Autodesk Inventor part; units mm, degrees
ref_plane "YZ Plane" through (0, 0, 0) normal (1, 0, 0) x (0, 1, 0)
ref_plane "XZ Plane" through (0, 0, 0) normal (0, 1, 0) x (-1, 0, 0)
ref_plane "XY Plane" through (0, 0, 0) normal (0, 0, 1) x (1, 0, 0)
sketch "Sketch1" plane through (0, 0, 0) normal (0, 1, 0) x (-1, 0, 0)
  line L0 (52.5, 37) -> (-52.5, 37)
  line L1 (-54.5, 35) -> (-54.5, -35)
  line L2 (-52.5, -37) -> (52.5, -37)
  line L3 (54.5, -35) -> (54.5, 35)
  line L4 (54.5, 37) -> (-54.5, -37) construction
  line L5 (-54.5, 37) -> (54.5, -37) construction
  circle A0 centre (-40.5, -31) radius 2.15
  circle A1 centre (-40.5, 31) radius 2.15
  circle A2 centre (9.5, -31) radius 2.15
  circle A3 centre (9.5, 31) radius 2.15
  circle A4 centre (32.1, 26) radius 2.15
  circle A5 centre (32.1, -26) radius 2.15
  circle A6 centre (9.6, 12.319) radius 3.95
  circle A7 centre (9.6, -12.319) radius 3.95
  circle A8 centre (-40.4, 12.319) radius 3.95
  circle A9 centre (-40.4, -12.319) radius 3.95
  circle A10 centre (43.1, 19.95) radius 3.95
  circle A11 centre (43.1, -19.95) radius 3.95
  arc A12 (54.5, 35) -> (52.5, 37) centre (52.5, 35) ccw
  arc A13 (52.5, -37) -> (54.5, -35) centre (52.5, -35) ccw
  arc A14 (-54.5, -35) -> (-52.5, -37) centre (-52.5, -35) ccw
  arc A15 (-52.5, 37) -> (-54.5, 35) centre (-52.5, 35) ccw
  circle A16 centre (44.5, -7.5) radius 2
  circle A17 centre (44.5, 7.5) radius 2
  point P0 (0, 0)
  dimension "d0" = 109
  dimension "d1" = 74
  dimension "d2" = 4.3
  dimension "d3" = 6
  dimension "d4" = 14
  dimension "d5" = 4.3
  dimension "d6" = 6
  dimension "d7" = 14
  dimension "d8" = 4.3
  dimension "d9" = 6
  dimension "d10" = 64
  dimension "d11" = 4.3
  dimension "d12" = 6
  dimension "d13" = 64
  dimension "d14" = 4.3
  dimension "d20" = 7.9
  dimension "d22" = 7.9
  dimension "d24" = 64.1
  dimension "d25" = 64.1
  dimension "d26" = 7.9
  dimension "d27" = 50
  dimension "d28" = 24.638
  dimension "d29" = 12.319
  dimension "d30" = 12.319
  dimension "d31" = 7.9
  dimension "d32" = 24.638
  dimension "d33" = 50
  dimension "d34" = 7.9
  dimension "d35" = 7.9
  dimension "d36" = 39.9
  dimension "d37" = 19.95
  dimension "d42" = 2
  dimension "d59" = 11
  dimension "d61" = 26
  dimension "d63" = 52
  dimension "d64" = 11
  dimension "d65" = 4.3
  dimension "d66" = 33.5
  dimension "d67" = 33.5
  dimension "d70" = 4
  dimension "d71" = 4
  dimension "d72" = 15
  dimension "d73" = 7.5
  dimension "d74" = 10
  dimension "d75" = 10
extrude "Extrusion5" add sketch "Sketch1" along normal blind 5
thread "Thread1"
thread "Thread2"
sketch "Sketch2" plane through (0, 5, 0) normal (0, 1, 0) x (1, 0, 0)
  line L0 (-54.5, 30) -> (-45.5, 30)
  line L1 (-45.5, 30) -> (-45.5, 37)
  line L2 (-54.5, 35) -> (-54.5, -35)
  line L3 (52.5, 37) -> (-52.5, 37)
  line L4 (-45.5, -37.1799) -> (-45.5, -30.1799)
  line L5 (-45.5, -30.1799) -> (-54.5, -30.1799)
  line L6 (-54.5, 30) -> (-54.5, 37)
  line L7 (-54.5, 37) -> (-45.5, 37)
  line L8 (-45.5, -37.1799) -> (-54.5, -37.1799)
  line L9 (-54.5, -37.1799) -> (-54.5, -30.1799)
  point P0 (0, 0)
  dimension "d84" = 9
  dimension "d85" = 7
  dimension "d86" = 7
extrude "Extrusion7" cut sketch "Sketch2" against normal blind 10
fillet "Fillet1" radius 2 8 edges at (-50, 5, 30.1799) (-45.5, 5, 33.59) (-50, 5, -30) (-45.5, 5, -33.5) (-50, 0, 30.1799) (-45.5, 0, 33.59) (-50, 0, -30) (-45.5, 0, -33.5)
equation "\"d86\" = d85"
properties part number "TopSupport"
For this review, take the finished solid that the model builds, in its own axes (mm). A direction names the side the tool comes from. Round coordinates to 2 decimals unless told otherwise and drop trailing zeros. Loops run counter-clockwise (first coordinate to the right, second up) from the corner with the lowest first, then second, coordinate; pieces in that order, holes last. Notation, with made-up numbers: (-10.5, 27.25) - (14.5, 27.25) arc R18 cw to (14.5, 53.25) - close; hole circle Ø4 at (83, 78.5). An arc over 180 degrees is marked (long way). Put each result on its own line as item: value. Start each with the question number.
1. Consider section B-B on x = -9.6. State the section outline as (y, z) points.
2. Consider section A-A on z = 19.95. State the section outline as (x, y) points.
3. For faces 1 (the cylindrical face through (-29.95, 2.46, -26.09)), 2 (the cylindrical face through (-49.08, 4.4, 29.61)), 3 (the flat face through (1, 0, 1)), 4 (the cylindrical face through (-44.93, 4.4, -33.56)), 5 (the cylindrical face through (-44.9, 0.57, 33.51)), list the 3-axis set-ups (+Z, -Z, +X, -X, +Y, -Y) from which the entire face can be reached by the end or side of a thin tool; tool diameter is ignored.
4. Consider section D-D on y = 0.75. State how many separate pieces and enclosed holes the cut face has, plus the area to 3 significant figures.
5. For probe 1 along Z at (x, y) = (-32.1, 1.4); probe 2 along Z at (x, y) = (-9.5, 2.85); probe 3 along X at (y, z) = (2.4, -9), list the stretches that pass through material, from the lowest coordinate up. Write a range as [from, to].
6. Insertion check: P1, Ø1.1, axis at y = 2.5, z = 35, coming from the -X side; P2, Ø0.8, axis at x = -49, y = 2.5, coming from the +Z side. Each pin has a flat end and moves straight along its axis. Give the tip position at first contact, or say it passes through.
7. Consider section C-C on x = -32.1. State the section outline as (y, z) points, plus the area to 3 significant figures.
Result sheet:
1. outline: (0, -37) - (5, -37) - (5, -33.15) - (0, -33.15) - close; (0, -28.85) - (5, -28.85) - (5, -16.27) - (0, -16.27) - close; (0, -8.37) - (5, -8.37) - (5, 8.37) - (0, 8.37) - close; (0, 16.27) - (5, 16.27) - (5, 28.85) - (0, 28.85) - close; (0, 33.15) - (5, 33.15) - (5, 37) - (0, 37) - close
2. outline: (-54.5, 0) - (-47.05, 0) - (-47.05, 5) - (-54.5, 5) - close; (-39.15, 0) - (54.5, 0) - (54.5, 5) - (-39.15, 5) - close
3. face 1: +Y, -Y
3. face 2: +Z, -X, +Y
3. face 3: +Z, -Z, +X, -X, -Y
3. face 4: -Z, -X, +Y
3. face 5: +Z, -X, -Y
4. separate pieces: 1
4. enclosed holes: 14
4. area: 7,520 mm^2
5. probe 1: [-37, -28.15], [-23.85, 23.85], [28.15, 37]
5. probe 2: [-37, -33.15], [-28.85, -16.27], [-8.37, 8.37], [16.27, 28.85], [33.15, 37]
5. probe 3: [-54.5, -45.82], [-43.18, -11.74], [-7.46, 38.26], [42.54, 54.5]
6. P1: x = -45.5
6. P2: z = 30.18
7. outline: (0, -37) - (5, -37) - (5, -28.15) - (0, -28.15) - close; (0, -23.85) - (5, -23.85) - (5, 23.85) - (0, 23.85) - close; (0, 28.15) - (5, 28.15) - (5, 37) - (0, 37) - close
7. area: 327 mm^2
